For this review, use the dimensioned drawing (mm, ordinates from the lowest corner) and the shaded views. Round coordinates to 2 decimals unless told otherwise and drop trailing zeros. Write each loop counter-clockwise with the first axis right and the second up, starting at its lowest first coordinate (ties: lowest second). Pieces come first, ordered by that corner, then holes. Notation, with made-up numbers: (-39, -4.75) - (-7, -4.75) arc R23 ccw to (-7, 19.25) - close; hole circle Ø10 at (-10, 19). An arc over 180 degrees is marked (long way). Write each question's results on one line, items separated by ' | '.
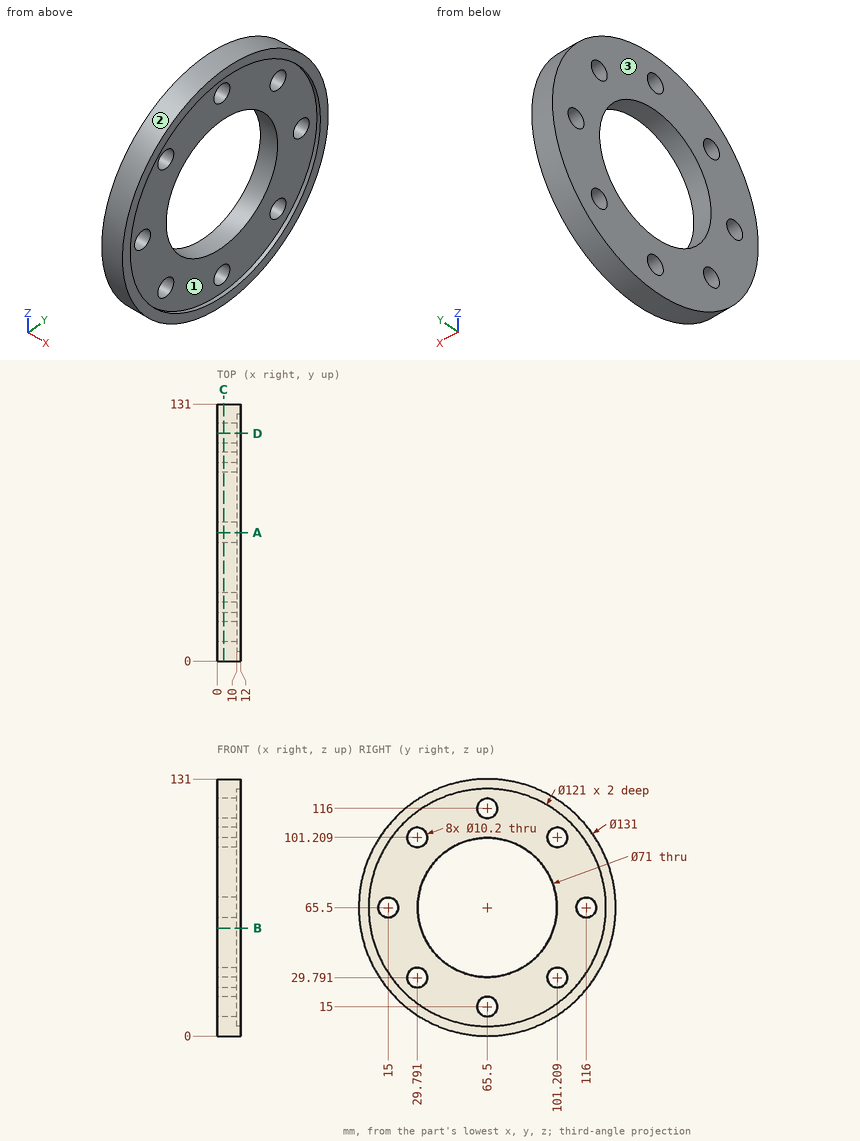
Q1. We need section D-D (y = 116). State the section outline as (x, z) points.
Evaluation:
outline: (0, 23.79) - (12, 23.79) - (12, 32.18) - (10, 32.18) - (10, 60.4) - (0, 60.4) - close; (0, 70.6) - (10, 70.6) - (10, 98.82) - (12, 98.82) - (12, 107.21) - (0, 107.21) - close
Q2. For probe 1 along Z at (x, y) = (8.75, 66); probe 2 along Z at (x, y) = (5, 34); probe 3 along Y at (x, z) = (11.05, 65.5), list the stretches that pass through material, from the lowest coordinate up.
Evaluation:
probe 1: z = 0 to 9.92, 20.08 to 30, 101 to 110.92, 121.08 to 131 | probe 2: z = 8.07 to 26.91, 32.67 to 49.13, 81.87 to 98.33, 104.09 to 122.93 | probe 3: y = 0 to 5, 126 to 131
Q3. Insertion check: P1, Ø4, axis at x = 4, z = 61.5, coming from the -Y side; P2, Ø6, axis at x = 3.5, z = 58.5, coming from the +Y side; P3, Ø5, axis at y = 94.5, z = 48, coming from the +X side. Each pin has a flat end and moves straight along its axis. Give the tip position at first contact, or say it passes through.
Evaluation:
P1: stops at y = 0.03 | P2: stops at y = 130.88 | P3: stops at x = 10
Q4. We need section A-A (y = 65.5). State the section outline as (x, z) points.
Evaluation:
outline: (0, 0) - (12, 0) - (12, 5) - (10, 5) - (10, 9.9) - (0, 9.9) - close; (0, 20.1) - (10, 20.1) - (10, 30) - (0, 30) - close; (0, 101) - (10, 101) - (10, 110.9) - (0, 110.9) - close; (0, 121.1) - (10, 121.1) - (10, 126) - (12, 126) - (12, 131) - (0, 131) - close
Q5. We need section B-B (z = 55). State the section outline as (x, y) points, plus the area to 3 significant figures.
Evaluation:
outline: (0, 0.85) - (12, 0.85) - (12, 5.92) - (10, 5.92) - (10, 31.59) - (0, 31.59) - close; (0, 99.41) - (10, 99.41) - (10, 125.08) - (12, 125.08) - (12, 130.15) - (0, 130.15) - close | area: 635 mm^2
Q6. The part is to be moulded in two halves that separate along Z. For the marked faces 1, 2 and 3, say which applies: released by +Z, released by -Z, zero draft, split by the parting line, or undercut.
Evaluation:
face 1: undercut | face 2: split by the parting line | face 3: zero draft
Q7. We need section C-C (x = 3.25). State how many separate pieces and enclosed holes the cut face has, plus the area to 3 significant figures.
Evaluation:
separate pieces: 1 | enclosed holes: 9 | area: 8,870 mm^2
